from build123d import *

# Parameters (mm, degrees)
RESSALTO_EXTRUS_O1_DEPTH = 25
FILETE1_R                = 1.5
CORTE_EXTRUS_O1_REACH    = 35.483
ESBO_O3_W                = 4
ESBO_O3_H                = 2.5
FILETE2_R                = 1
FILETE3_R                = 3


with BuildPart() as part:
    # Esboço1 → Ressalto-extrusão1 (new body)
    with BuildSketch(Plane.XY):
        with BuildLine():
            Line((-17, 10.5), (17, 10.5))
            Line((17, 10.5), (17, 7.5))
            Line((17, 7.5), (9, 7.5))
            Line((9, 7.5), (9, 5.408326913))
            ThreePointArc((9, 5.408326913), (10.485597072, 0.549776353), (9.516231764, -4.437491748))
            Line((9.516231764, -4.437491748), (7.650118208, -3.567308706))
            ThreePointArc((7.650118208, -3.567308706), (7.15483055, -3.057799008), (7.123002767, -2.347941987))
            ThreePointArc((7.123002767, -2.347941987), (0, 7.5), (-7.123002767, -2.347941987))
            ThreePointArc((-7.123002767, -2.347941987), (-7.15483055, -3.057799008), (-7.650118208, -3.567308706))
            Line((-7.650118208, -3.567308706), (-9.516231764, -4.437491748))
            ThreePointArc((-9.516231764, -4.437491748), (-10.485597072, 0.549776353), (-9, 5.408326913))
            Line((-9, 5.408326913), (-9, 7.5))
            Line((-9, 7.5), (-17, 7.5))
            Line((-17, 7.5), (-17, 10.5))
        make_face()
    extrude(amount=RESSALTO_EXTRUS_O1_DEPTH)

    # Filete1
    filete1_edges = [part.edges().sort_by_distance(p)[0] for p in [
        (-9.516231764, -4.437491748, 12.5),
        (9.516231764, -4.437491748, 12.5),
    ]]
    fillet(filete1_edges, radius=FILETE1_R)

    # Esboço3 → Corte-extrusão1 (cut, up to next)
    with BuildSketch(Plane(origin=(0, 10.5, 0), x_dir=(1, 0, 0), z_dir=(0, 1, 0)), mode=Mode.PRIVATE) as corte_extrus_o1_sk1:
        with Locations((-12.5, -4.25)):
            Rectangle(ESBO_O3_W, ESBO_O3_H)
    corte_extrus_o1_tool1 = extrude(corte_extrus_o1_sk1.sketch, amount=-CORTE_EXTRUS_O1_REACH, mode=Mode.PRIVATE) & part.part
    # Esboço3 → Corte-extrusão1 (cut, up to next)
    with BuildSketch(Plane(origin=(0, 10.5, 0), x_dir=(1, 0, 0), z_dir=(0, 1, 0)), mode=Mode.PRIVATE) as corte_extrus_o1_sk2:
        with Locations((-12.5, -20.75)):
            Rectangle(ESBO_O3_W, ESBO_O3_H)
    corte_extrus_o1_tool2 = extrude(corte_extrus_o1_sk2.sketch, amount=-CORTE_EXTRUS_O1_REACH, mode=Mode.PRIVATE) & part.part
    # Esboço3 → Corte-extrusão1 (cut, up to next)
    with BuildSketch(Plane(origin=(0, 10.5, 0), x_dir=(1, 0, 0), z_dir=(0, 1, 0)), mode=Mode.PRIVATE) as corte_extrus_o1_sk3:
        with Locations((12.5, -20.75)):
            Rectangle(ESBO_O3_W, ESBO_O3_H)
    corte_extrus_o1_tool3 = extrude(corte_extrus_o1_sk3.sketch, amount=-CORTE_EXTRUS_O1_REACH, mode=Mode.PRIVATE) & part.part
    # Esboço3 → Corte-extrusão1 (cut, up to next)
    with BuildSketch(Plane(origin=(0, 10.5, 0), x_dir=(1, 0, 0), z_dir=(0, 1, 0)), mode=Mode.PRIVATE) as corte_extrus_o1_sk4:
        with Locations((12.5, -4.25)):
            Rectangle(ESBO_O3_W, ESBO_O3_H)
    corte_extrus_o1_tool4 = extrude(corte_extrus_o1_sk4.sketch, amount=-CORTE_EXTRUS_O1_REACH, mode=Mode.PRIVATE) & part.part
    add(corte_extrus_o1_tool1.solids().sort_by_distance((-12.5, 10.5, 4.25))[0], mode=Mode.SUBTRACT)
    add(corte_extrus_o1_tool2.solids().sort_by_distance((-12.5, 10.5, 20.75))[0], mode=Mode.SUBTRACT)
    add(corte_extrus_o1_tool3.solids().sort_by_distance((12.5, 10.5, 20.75))[0], mode=Mode.SUBTRACT)
    add(corte_extrus_o1_tool4.solids().sort_by_distance((12.5, 10.5, 4.25))[0], mode=Mode.SUBTRACT)

    # Filete2
    filete2_edges = [part.edges().sort_by_distance(p)[0] for p in [
        (12.5, 10.5, 5.5),
        (12.5, 7.5, 5.5),
        (12.5, 10.5, 19.5),
        (12.5, 7.5, 19.5),
        (-12.5, 10.5, 19.5),
        (-12.5, 7.5, 19.5),
        (-12.5, 10.5, 5.5),
        (-12.5, 7.5, 5.5),
    ]]
    fillet(filete2_edges, radius=FILETE2_R)

    # Filete3
    filete3_edges = [part.edges().sort_by_distance(p)[0] for p in [
        (-17, 9, 0),
        (17, 9, 0),
        (17, 9, 25),
        (-17, 9, 25),
    ]]
    fillet(filete3_edges, radius=FILETE3_R)


solid = part.part
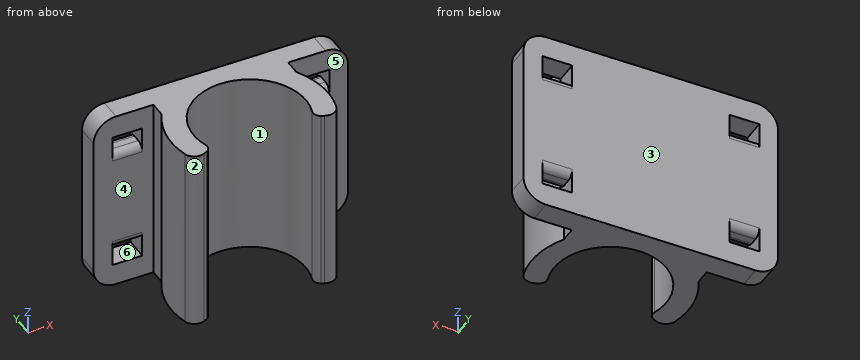
The model under review builds one solid part; all positions refer to its coordinate system, in mm. Face numbers are marked on the shaded views. A direction names the side the tool comes from. Round coordinates to 2 decimals unless told otherwise and drop trailing zeros. Order: outer loops, then holes, each group sorted by start corner. A loop starts at its lowest first (then second) coordinate and runs counter-clockwise, first axis right, second up. Notation, with made-up numbers: (50, 7.5) -> (68, 7.5) arc R17 ccw to (68, 11.5) -> close; hole circle Ø5 at (6.5, 74.25). An arc over 180 degrees is marked (long way). Return JSON: item names as keys, results as strings.
1. Take a section at D-D (x = 0). Write out the cut boundary in (y, z), then the cut area to 3 significant figures.
Answer block:
{"outline": "(7.5, 0) -> (10.5, 0) -> (10.5, 25) -> (7.5, 25) -> close", "area": "75.0 mm²"}
2. Take a section at C-C (z = 14.25). Write out the cut boundary in (x, y).
Answer block:
{"outline": "(-17, 7.5) -> (-9, 7.5) -> (-9, 5.41) arc R10.5 ccw to (-10.12, -2.79) arc R1.5 ccw to (-8.04, -3.75) -> (-7.65, -3.57) arc R1 ccw to (-7.12, -2.35) arc R7.5 cw (long way) to (7.12, -2.35) arc R1 ccw to (7.65, -3.57) -> (8.04, -3.75) arc R1.5 ccw to (10.12, -2.79) arc R10.5 ccw to (9, 5.41) -> (9, 7.5) -> (17, 7.5) -> (17, 10.5) -> (-17, 10.5) -> close"}
3. Take a section at B-B (y = 8). Write out the cut boundary in (x, z).
Answer block:
{"outline": "(-17, 3) arc R3 ccw to (-14, 0) -> (14, 0) arc R3 ccw to (17, 3) -> (17, 22) arc R3 ccw to (14, 25) -> (-14, 25) arc R3 ccw to (-17, 22) -> close; hole (-14.5, 3) -> (-10.5, 3) -> (-10.5, 5.63) -> (-14.5, 5.63) -> close; hole (-14.5, 19.37) -> (-10.5, 19.37) -> (-10.5, 22) -> (-14.5, 22) -> close; hole (10.5, 3) -> (14.5, 3) -> (14.5, 5.63) -> (10.5, 5.63) -> close; hole (10.5, 19.37) -> (14.5, 19.37) -> (14.5, 22) -> (10.5, 22) -> close"}
4. Take a section at A-A (y = 0). Write out the cut boundary in (x, z), then the cut area to 3 significant figures.
Answer block:
{"outline": "(-10.5, 0) -> (-7.5, 0) -> (-7.5, 25) -> (-10.5, 25) -> close; (7.5, 0) -> (10.5, 0) -> (10.5, 25) -> (7.5, 25) -> close", "area": "150 mm²"}
5. For the marked faces 4, 5 and 6, list the 3-axis set-ups (+Z, -Z, +X, -X, +Y, -Y) from which the entire face can be reached by the end or side of a thin tool; tool diameter is ignored.
Answer block:
{"face 4": "+Z, -Z, -X", "face 5": "+Z, -Z, +X", "face 6": "+Y, -Y"}
6. The part is to be moulded in two halves that separate along Y. For the marked faces 1, 2 and 3, say which applies: +Y half, -Y half, draft (parallel to the pull), parting line (faces both ways), or undercut.
Answer block:
{"face 1": "undercut", "face 2": "-Y half", "face 3": "+Y half"}
7. Insertion check: P1, Ø5, axis at x = 8.5, y = -0.5, coming from the -Z side; P2, Ø1.5, axis at x = -11.5, z = 10, coming from the -Y side; P3, Ø1, axis at y = 6, z = 10, coming from the -X side; P4, Ø2, axis at y = 3.5, z = 19.5, coming from the +X side. Each pin has a flat end and moves straight along its axis. Give the tip position at first contact, or say it passes through.
Answer block:
{"P1": "stops at z = 0", "P2": "stops at y = 7.5", "P3": "stops at x = -9", "P4": "stops at x = 10.2"}
8. For L1, parallel to X at y = 9.25, z = 21.75; L2, parallel to X at y = 0, z = 6.75; L3, parallel to X at y = 1.25, z = 11.75, list the stretches that pass through material, from the lowest coordinate up. Write a range as [from, to].
Answer block:
{"L1": "x = [-17, -14.5], [-10.5, 10.5], [14.5, 17]", "L2": "x = [-10.5, -7.5], [7.5, 10.5]", "L3": "x = [-10.43, -7.4], [7.4, 10.43]"}
